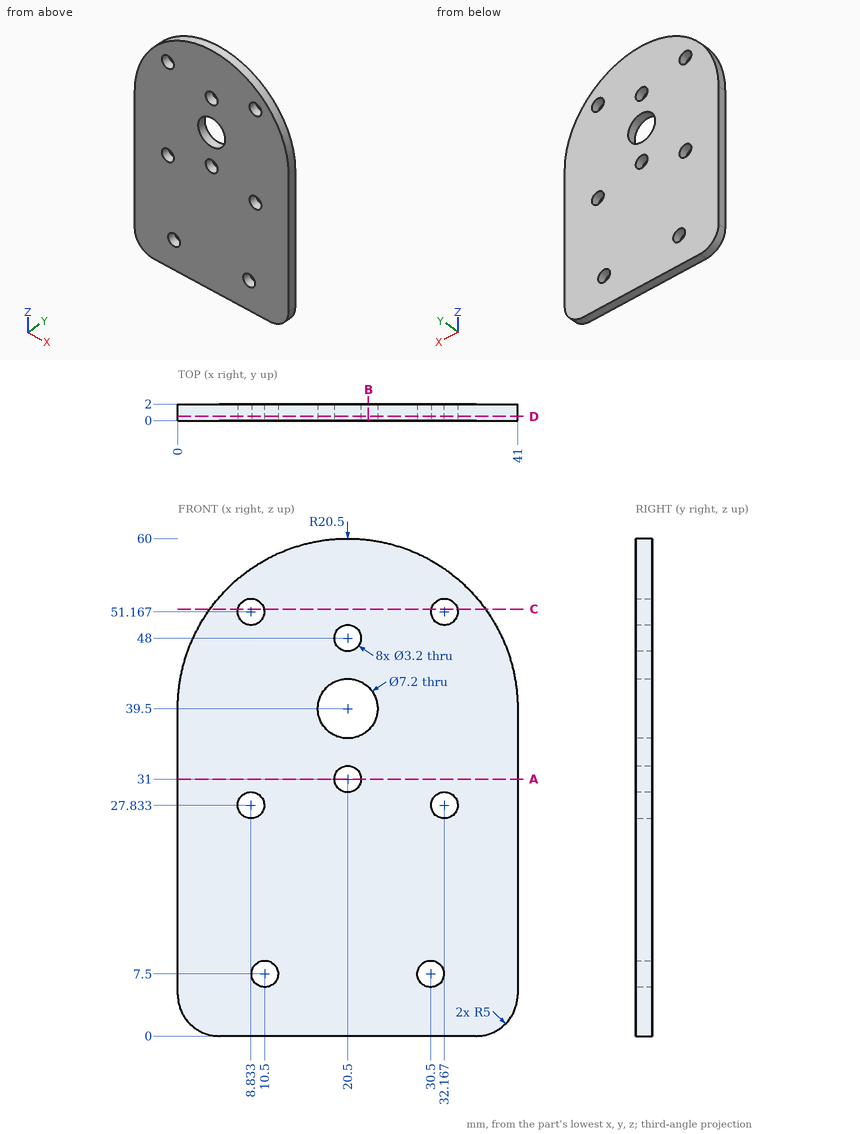
The drawing under review shows one solid part. Ordinate dimensions are in mm from its lowest x, y, z. Round coordinates to 2 decimals unless told otherwise and drop trailing zeros. Write each loop counter-clockwise with the first axis right and the second up, starting at its lowest first coordinate (ties: lowest second). Pieces come first, ordered by that corner, then holes. Notation, with made-up numbers: M 70,34.5 L 84,34.5 A21 ccw 84,39.5 Z; hole C 40,80 d1. An arc over 180 degrees is marked long. One line per item, written item: value. Start each with the question number.
(1) We need section A-A (z = 31). Give the boundary of the cut face in (x, y), and give its area (3 significant figures).
(2) We need section D-D (y = 0.5). Count the separate pieces of the cut face and the enclosed holes in it, and give its area (3 significant figures).
(3) Wall thickness on line 1 (Z direction, x = 7.5, y = 0.8); line 2 (X direction, y = 1.2, z = 31); line 3 (X direction, y = 0.5, z = 36.5): over which ranges is each line inside the solid? List them lowest first.
(4) We need section B-B (x = 23). Give the boundary of the cut face in (y, z), and give its area (3 significant figures).
(5) We need section C-C (z = 51.5). Give the boundary of the cut face in (x, y).
Result:
1. outline: M 0,0 L 18.9,0 L 18.9,2 L 0,2 Z; M 22.1,0 L 41,0 L 41,2 L 22.1,2 Z
1. area: 75.6 mm²
2. separate pieces: 1
2. enclosed holes: 9
2. area: 2,160 mm²
3. line 1: 0 to 26.95, 28.72 to 50.28, 52.05 to 55.35
3. line 2: 0 to 18.9, 22.1 to 41
3. line 3: 0 to 18.51, 22.49 to 41
4. outline: M 0,0 L 2,0 L 2,36.91 L 0,36.91 Z; M 0,42.09 L 2,42.09 L 2,59.85 L 0,59.85 Z
4. area: 109 mm²
5. outline: M 3.88,0 L 7.27,0 L 7.27,2 L 3.88,2 Z; M 10.4,0 L 30.6,0 L 30.6,2 L 10.4,2 Z; M 33.73,0 L 37.12,0 L 37.12,2 L 33.73,2 Z
